Autodesk Inventor part; units mm, degrees
ref_plane "YZ Plane" through (0, 0, 0) normal (1, 0, 0) x (0, 1, 0)
ref_plane "XZ Plane" through (0, 0, 0) normal (0, 1, 0) x (-1, 0, 0)
ref_plane "XY Plane" through (0, 0, 0) normal (0, 0, 1) x (1, 0, 0)
sketch "Esquisse1" plane through (0, 0, 0) normal (0, 1, 0) x (-1, 0, 0)
  line L0 (0, -6.7291) -> (0, 2.2709)
  line L1 (0, 2.2709) -> (-5, 2.2709)
  line L2 (-5, 2.2709) -> (-5, -3.2291)
  line L3 (-5, -3.2291) -> (-7.5, -3.2291)
  line L4 (0, -6.7291) -> (-7.5, -6.7291)
  line L5 (-7.5, -3.2291) -> (-7.5, -6.7291)
  point P0 (0, 0)
  dimension "d0" = 9
  dimension "d1" = 5
  dimension "d2" = 5.5
  dimension "d3" = 7.5
revolve "Révolution1" add sketch "Esquisse1" angle 360 about axis through (0, 0, -6.7291) along (0, 0, 1)
fillet "Congé1" radius 2 1 edges at (-7.5, 0, -6.7291)
fillet "Congé2" radius 0.5 1 edges at (-7.5, 0, -3.2291)
fillet "Congé3" radius 0.5 1 edges at (-5, 0, -3.2291)
hole "Perçage1" at (0, 0, 2.2709) direction (0, 0, -1) diameter 2.5 depth 7
properties part number "pied" material "Plastique ABS"
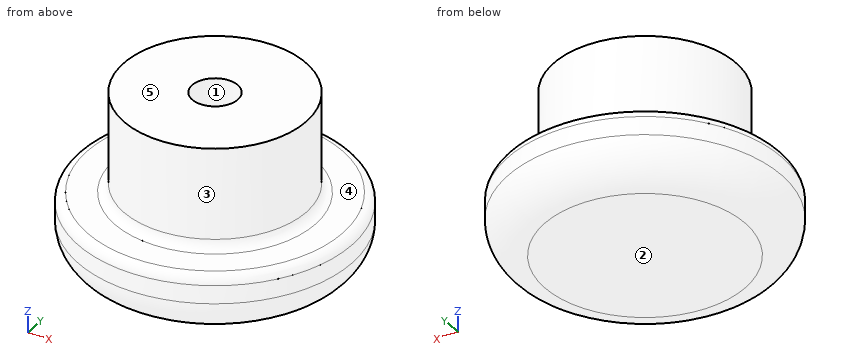
Geometry: final body of the model. Coordinates: model frame, mm. Face numbers are marked on the shaded views. A direction names the side the tool comes from. Coordinates: 2 decimals unless noted, no trailing zeros. Order: outer loops, then holes, each group sorted by start corner. A loop starts at its lowest first (then second) coordinate and runs counter-clockwise, first axis right, second up. Notation, with made-up numbers: (-11.5, 9.25) - (2.5, 9.25) arc R18 ccw to (2.5, 18.25) - close; hole circle Ø10 at (-17.5, 23.25). An arc over 180 degrees is marked (long way). Use one line per item in the form item = value.
1) Section A-A (x = 0). Return loops of the section in (y, z).
Solutions:
outline = (-7.5, -4.73) arc R2 ccw to (-5.5, -6.73) - (5.5, -6.73) arc R2 ccw to (7.5, -4.73) - (7.5, -3.73) arc R0.5 ccw to (7, -3.23) - (5.5, -3.23) arc R0.5 cw to (5, -2.73) - (5, 2.27) - (1.25, 2.27) - (1.25, -4.73) - (-1.25, -4.73) - (-1.25, 2.27) - (-5, 2.27) - (-5, -2.73) arc R0.5 cw to (-5.5, -3.23) - (-7, -3.23) arc R0.5 ccw to (-7.5, -3.73) - close
2) Pin query (flat end, axial travel): pin 1 (3 mm diameter, centred on x = 3, z = -3, fed in from +Y); pin 2 (4 mm diameter, centred on x = 5.5, z = -1.5, fed in from +Y); pin 3 (1.5 mm diameter, centred on x = 0, y = 0, fed in from +Z). Return the tip coordinate at first contact, or that it passes through.
Solutions:
pin_1 = 7.31
pin_2 = 5.59
pin_3 = -4.73
3) Section D-D (z = 1). Return loops of the section in (x, y), then the cut area to 3 significant figures.
Solutions:
outline = circle Ø10 at (0, 0); hole circle Ø2.5 at (0, 0)
area = 73.6 mm^2
4) Section C-C (z = -4). Return loops of the section in (x, y), then the cut area to 3 significant figures.
Solutions:
outline = circle Ø15 at (0, 0); hole circle Ø2.5 at (0, 0)
area = 172 mm^2
5) Mould query, pull axis Y, two halves, no side actions, for the marked faces 1, 2 and 3. Classes: +Y half, -Y half, draft (parallel to the pull), parting line (faces both ways), or undercut.
Solutions:
face_1 = undercut
face_2 = draft
face_3 = parting line
6) Ray query, L1, parallel to Y at x = 0, z = -2.75; L2, parallel to X at y = -0.5, z = -2.25; L3, parallel to Y at x = -3, z = -0.5. Return the intervals inside material, ascending.
Solutions:
L1 = -5 to -1.25, 1.25 to 5
L2 = -4.97 to -1.15, 1.15 to 4.97
L3 = -4 to 4
7) Set-up query: the marked faces 4 and 5. Return all of +Z, -Z, +X, -X, +Y, -Y with unobstructed straight access to the full face (end or side cutting, diameter ignored); none if empty.
Solutions:
face_4 = +Z
face_5 = +Z, +X, -X, +Y, -Y
